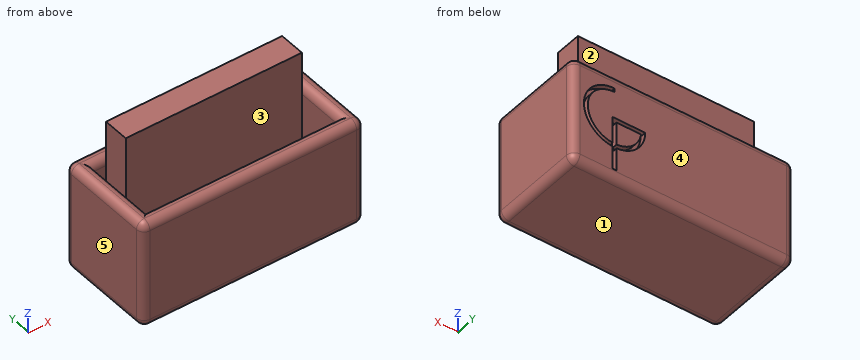
```python
from build123d import *

# Parameters (mm, degrees)
F0_W     = 14.5
F0_H     = 6.6
F0_W_2   = 12.5
F0_H_2   = 4.6
F1_DEPTH = 7
F0_W_3   = 11.5
F0_H_3   = 1.7
F2_DEPTH = 2
F3_DEPTH = 10
F5_DEPTH = 0.4
F6_R     = 0.49999


# Not quite as in the source:
# - a fillet or chamfer is up to 0.001 mm smaller than in the source, because OpenCascade refuses the exact size


with BuildPart() as f1:
    # F0 (on Top) → F1 (new body)
    with BuildSketch(Plane.XY):
        with Locations((0.6113282288, 0)):
            Rectangle(F0_W, F0_H)
        with Locations((0.6113282288, 0)):
            Rectangle(F0_W_2, F0_H_2, mode=Mode.SUBTRACT)
    extrude(amount=F1_DEPTH)

    # F0 (on Top) → F2 (join)
    with BuildSketch(Plane.XY):
        with Locations((0.6113282288, 0)):
            Rectangle(F0_W_2, F0_H_2)
        with Locations((0.6113282288, 0.95)):
            Rectangle(F0_W_3, F0_H_3, mode=Mode.SUBTRACT)
        with Locations((0.6113282288, 0.95)):
            Rectangle(F0_W_3, F0_H_3)
    extrude(amount=F2_DEPTH)

    # F0 (on Top) → F3 (join)
    with BuildSketch(Plane.XY):
        with Locations((0.6113282288, 0.95)):
            Rectangle(F0_W_3, F0_H_3)
    extrude(amount=F3_DEPTH)

    # F4 (on face) → F5 (cut)
    with BuildSketch(Plane(origin=(0, 3.3, 0), x_dir=(-1, 0, 0), z_dir=(0, 1, 0))):
        with BuildLine():
            Line((-5.1014683965, 5.8378594238), (-5.1014683965, 6.0878594238))
            ThreePointArc((-5.1014683965, 6.0878594238), (-7.1005673821, 4.1478864664), (-5.2214683965, 2.0914626697))
            Line((-5.2214683965, 2.0914626697), (-5.2214683965, 2.3419785573))
            ThreePointArc((-5.2214683965, 2.3419785573), (-6.8504383099, 4.1478947619), (-5.1014683965, 5.8378594238))
        make_face()
        with BuildLine():
            Line((-5.2214683965, 2.3419785573), (-5.2214683965, 2.0914626697))
            ThreePointArc((-5.2214683965, 2.0914626697), (-5.0964586021, 2.0878656984), (-4.9714683965, 2.0920888959))
            Line((-4.9714683965, 2.0920888959), (-4.9714683965, 2.3426946752))
            ThreePointArc((-4.9714683965, 2.3426946752), (-5.0964555923, 2.3378666033), (-5.2214683965, 2.3419785573))
        make_face()
        with BuildLine():
            ThreePointArc((-4.9714683965, 2.0920888959), (-5.0964586021, 2.0878656984), (-5.2214683965, 2.0914626697))
            Line((-5.2214683965, 2.0914626697), (-5.2214683965, 0.5878594238))
            Line((-5.2214683965, 0.5878594238), (-4.9714683965, 0.5878594238))
            Line((-4.9714683965, 0.5878594238), (-4.9714683965, 2.0920888959))
        make_face()
        with BuildLine():
            Line((-4.9714683965, 2.3426946752), (-4.9714683965, 2.0920888959))
            ThreePointArc((-4.9714683965, 2.0920888959), (-3.6420164446, 2.7203799907), (-3.1014683965, 4.0878594238))
            Line((-3.1014683965, 4.0878594238), (-3.3514683965, 4.0878594238))
            ThreePointArc((-3.3514683965, 4.0878594238), (-3.3559614625, 3.9625376644), (-3.3694175889, 3.8378594238))
            ThreePointArc((-3.3694175889, 3.8378594238), (-3.907446743, 2.8084797729), (-4.9714683965, 2.3426946752))
        make_face()
        with BuildLine():
            Line((-5.2214683965, 4.0878594238), (-5.2214683965, 2.3419785573))
            ThreePointArc((-5.2214683965, 2.3419785573), (-5.0964555923, 2.3378666033), (-4.9714683965, 2.3426946752))
            Line((-4.9714683965, 2.3426946752), (-4.9714683965, 3.8378594238))
            Line((-4.9714683965, 3.8378594238), (-3.3694175889, 3.8378594238))
            ThreePointArc((-3.3694175889, 3.8378594238), (-3.3559614625, 3.9625376644), (-3.3514683965, 4.0878594238))
            Line((-3.3514683965, 4.0878594238), (-5.2214683965, 4.0878594238))
        make_face()
    extrude(amount=-F5_DEPTH, mode=Mode.SUBTRACT)

    # F6 (radius 0.5 in the source; OpenCascade refuses exactly that, so slightly less here)
    f6_edges = [f1.edges().sort_by_distance(p)[0] for p in [
        (7.861328, 3.3, 3.5),
        (0.611328, 3.3, 7),
        (0.611328, 3.3, 0),
        (7.861328, 0, 0),
        (7.861328, 0, 7),
        (7.861328, -3.3, 3.5),
        (0.611328, -3.3, 0),
        (-6.638672, 0, 0),
        (-6.638672, 3.3, 3.5),
        (-6.638672, -3.3, 3.5),
        (0.611328, -3.3, 7),
        (-6.638672, 0, 7),
        (0.611328, 2.3, 7),
        (0.611328, -2.3, 7),
        (-5.638672, 0, 7),
        (6.861328, 0, 7),
    ]]
    fillet(f6_edges, radius=F6_R)


solid = f1.part
```
The listing builds one solid part. Answer for the finished solid, in the listing's coordinates (mm). Face numbers are marked on the shaded views. A direction names the side the tool comes from. Give positions to 0.01 mm unless a question says otherwise; leave off trailing zeros. Loops run counter-clockwise (first coordinate to the right, second up) from the corner with the lowest first, then second, coordinate; pieces in that order, holes last. Notation, with made-up numbers: (50, 35) - (55, 35) arc R20 cw to (55, 73) - close; hole circle Ø3 at (78.25, 2). An arc over 180 degrees is marked (long way). Return JSON: item names as keys, results as strings. Group by question number.
1. Which of the six approach directions +Z, -Z, +X, -X, +Y, -Y give full straight-line access (tool end or side, diameter ignored) to the marked faces 1 and 2?
2. Find section B-B (z = 3.25). Write down the section's boundary in (x, y), then the cut area to 3 significant figures.
3. Straight lines are drawn through the part: line 1 (Y direction, x = 5.5, z = 2.25); line 2 (X direction, y = 0.25, z = 3.25); line 3 (Y direction, x = -1.75, z = 6). For each, find the intervals that lie inside material, in ascending order. Write a range as [from, to].
4. Given pin 1 Ø1.5 at (x, z) = (3, 8.5) entering from +Y, flat-ended and moving along its own axis, determine where the tip first touches the part or whether it passes through.
5. Determine the mould class of the marked faces 3, 4 and 5 for opening direction Y: pulls with the +Y half, pulls with the -Y half, needs draft (parallel to the pull), parting line crosses it, or undercut.
6. Find section D-D (z = 4.25). Write down the section's boundary in (x, y), then the cut area to 3 significant figures.
Verdict:
{
 "1": {"face 1": "-Z, +X, -X, +Y, -Y", "face 2": "+Z"},
 "2": {"outline": "(-6.64, -2.8) arc R0.5 ccw to (-6.14, -3.3) - (7.36, -3.3) arc R0.5 ccw to (7.86, -2.8) - (7.86, 2.8) arc R0.5 ccw to (7.36, 3.3) - (6.92, 3.3) - (6.92, 2.9) - (6.64, 2.9) - (6.64, 3.3) - (5.22, 3.3) - (5.22, 2.9) - (4.97, 2.9) - (4.97, 3.3) - (3.57, 3.3) - (3.57, 2.9) - (3.29, 2.9) - (3.29, 3.3) - (-6.14, 3.3) arc R0.5 ccw to (-6.64, 2.8) - close; (-5.14, 0.1) - (6.36, 0.1) - (6.36, 1.8) - (-5.14, 1.8) - close; hole (-5.64, -2.3) - (6.86, -2.3) - (6.86, 2.3) - (-5.64, 2.3) - close", "area": "57.2 mm^2"},
 "3": {"line 1": "y = [-3.3, -2.3], [0.1, 1.8], [2.3, 2.9]", "line 2": "x = [-6.64, -5.64], [-5.14, 6.36], [6.86, 7.86]", "line 3": "y = [-3.3, -2.3], [0.1, 1.8], [2.3, 3.3]"},
 "4": {"pin 1": "stops at y = 1.8"},
 "5": {"face 3": "undercut", "face 4": "pulls with the +Y half", "face 5": "needs draft"},
 "6": {"outline": "(-6.64, -2.8) arc R0.5 ccw to (-6.14, -3.3) - (7.36, -3.3) arc R0.5 ccw to (7.86, -2.8) - (7.86, 2.8) arc R0.5 ccw to (7.36, 3.3) - (7.09, 3.3) - (7.09, 2.9) - (6.84, 2.9) - (6.84, 3.3) - (-6.14, 3.3) arc R0.5 ccw to (-6.64, 2.8) - close; (-5.14, 0.1) - (6.36, 0.1) - (6.36, 1.8) - (-5.14, 1.8) - close; hole (-5.64, -2.3) - (6.86, -2.3) - (6.86, 2.3) - (-5.64, 2.3) - close", "area": "57.4 mm^2"}
}
